Could you check a few things on this model? Use its own coordinates, in mm. Face numbers are marked on the shaded views. A direction names the side the tool comes from. Give positions to 0.01 mm unless a question says otherwise; leave off trailing zeros. Order: outer loops, then holes, each group sorted by start corner. A loop starts at its lowest first (then second) coordinate and runs counter-clockwise, first axis right, second up.
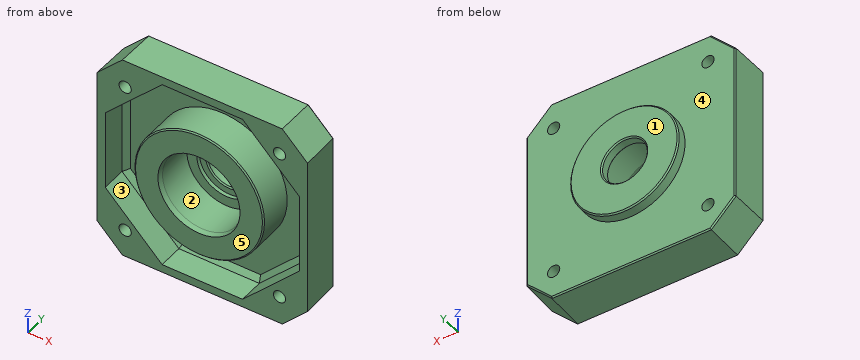
Autodesk Inventor part; units mm, degrees
ref_plane "YZ Plane" through (0, 0, 0) normal (1, 0, 0) x (0, 1, 0)
ref_plane "XZ Plane" through (0, 0, 0) normal (0, 1, 0) x (-1, 0, 0)
ref_plane "XY Plane" through (0, 0, 0) normal (0, 0, 1) x (1, 0, 0)
sketch "Sketch11" plane through (0, 0, 0) normal (0, 1, 0) x (-1, 0, 0)
  line L0 (-16, 21) -> (16, 21)
  line L1 (21, 16) -> (21, -16)
  line L2 (16, -21) -> (-16, -21)
  line L3 (-21, -16) -> (-21, 16)
  line L4 (-21, 21) -> (21, -21) construction
  line L5 (21, 21) -> (-21, -21) construction
  line L6 (21, -16) -> (16, -21)
  line L7 (-16, -21) -> (-21, -16)
  line L8 (-21, 16) -> (-16, 21)
  line L9 (16, 21) -> (21, 16)
  point P0 (0, 0)
  dimension "d82" = 42
  dimension "d83" = 5
  dimension "d84" = 5
  dimension "d85" = 5
  dimension "d86" = 5
  dimension "d87" = 5
  dimension "d88" = 5
  dimension "d89" = 5
  dimension "d90" = 5
extrude "Extrusion7" add sketch "Sketch11" against normal blind 8 draft 1
sketch "Sketch12" plane through (0, 0, 0) normal (0, 1, 0) x (1, 0, 0)
  circle A0 centre (0, 0) radius 10.9
  dimension "d93" = 21.8
extrude "Extrusion8" add sketch "Sketch12" along normal blind 2
sketch "Sketch13" plane through (0, -8, 0) normal (0, -1, 0) x (1, 0, 0)
  circle A0 centre (0, 0) radius 13
  line L0 (-8.0772, 19.5) -> (8.0772, 19.5)
  line L1 (8.0772, 19.5) -> (19.5, 8.0772)
  line L2 (19.5, 8.0772) -> (19.5, -8.0772)
  line L3 (19.5, -8.0772) -> (8.0772, -19.5)
  line L4 (8.0772, -19.5) -> (-8.0772, -19.5)
  line L5 (-8.0772, -19.5) -> (-19.5, -8.0772)
  line L6 (-19.5, -8.0772) -> (-19.5, 8.0772)
  line L7 (-19.5, 8.0772) -> (-8.0772, 19.5)
  dimension "d96" = 26
  dimension "d97" = 39
extrude "Extrusion9" cut sketch "Sketch13" against normal blind 6
sketch "Sketch14" plane through (0, -8, 0) normal (0, -1, 0) x (1, 0, 0)
  circle A0 centre (0, 0) radius 13
extrude "Extrusion10" add sketch "Sketch14" along normal blind 1
sketch "Sketch15" plane through (0, -9, 0) normal (0, -1, 0) x (1, 0, 0)
  circle A0 centre (0, 0) radius 8
  dimension "d102" = 16
extrude "Extrusion11" cut sketch "Sketch15" against normal blind 8.25
sketch "Sketch16" plane through (0, 2, 0) normal (0, 1, 0) x (1, 0, 0)
  point P0 (0, 0)
  point P1 (0, 0)
hole "Hole5" at (0, 2, 0) direction (0, -1, 0) diameter 9 end through all
sketch "Sketch17" plane through (0, -0.75, 0) normal (0, -1, 0) x (1, 0, 0)
  circle A0 centre (0, 0) radius 6
  dimension "d112" = 12
extrude "Extrusion12" cut sketch "Sketch17" against normal blind 0.75
sketch "Sketch18" plane through (0, 0, 0) normal (0, 1, 0) x (1, 0, 0)
  line L0 (-15.5, 15.5) -> (15.5, 15.5) construction
  line L1 (15.5, 15.5) -> (15.5, -15.5) construction
  line L2 (15.5, -15.5) -> (-15.5, -15.5) construction
  line L3 (-15.5, -15.5) -> (-15.5, 15.5) construction
  line L4 (-15.5, 15.5) -> (15.5, -15.5) construction
  line L5 (15.5, 15.5) -> (-15.5, -15.5) construction
  point P0 (0, 0)
  point P1 (0, 0)
  dimension "d115" = 31
  dimension "d124" = 31
hole "Hole6" at (-15.5, 0, -15.5) at (15.5, 0, -15.5) at (15.5, 0, 15.5) at (-15.5, 0, 15.5) direction (0, -1, 0) diameter 2.459 end through all
chamfer "Chamfer1" distance 0.25 distance2 1 1 edges at (-8, -9, 0) measured on face at (11.1299, -9, -1.6752)
chamfer "Chamfer2" distance 0.25 angle 45 12 edges at (-13, -9, 0) (0, 0, -4.5) (0, 2, -4.5) (-10.9, 2, 0) (-21, 0, 0) (-18.5, 0, 18.5) (0, 0, 21) (18.5, 0, 18.5) (21, 0, 0) (18.5, 0, -18.5) (0, 0, -21) (-18.5, 0, -18.5)
chamfer "Chamfer3" distance 1 angle 45 8 edges at (-13.7886, -2, -13.7886) (-19.5, -2, 0) (-13.7886, -2, 13.7886) (0, -2, 19.5) (13.7886, -2, 13.7886) (19.5, -2, 0) (13.7886, -2, -13.7886) (0, -2, -19.5)
equation "\"d84\" = d83"
equation "\"d85\" = d83"
equation "\"d86\" = d85"
equation "\"d87\" = d83"
equation "\"d88\" = d87"
equation "\"d89\" = d83"
equation "\"d90\" = d89"
properties part number "Nema 17 Top Cap" material "Aluminum 6061"
Item 1: For pin 1 (4 mm diameter, centred on x = -3.5, y = -2, fed in from +Z); pin 2 (1.5 mm diameter, centred on x = -8, y = -7, fed in from -Z); pin 3 (2 mm diameter, centred on x = 4.5, y = -0.5, fed in from -Z), each with a flat end and sliding along its axis, tell me the tip position at first contact or that it passes through.
Findings:
pin 1: stops at z = 21.07
pin 2: stops at z = -21.14
pin 3: stops at z = -21.03
Item 2: We'd pull the mould along Z, two halves only. Please class the marked faces 1 and 2: +Z half, -Z half, draft (parallel to the pull), parting line (faces both ways), or undercut.
Findings:
face 1: draft
face 2: undercut
Item 3: Imagine slicing it at B-B on y = -4. List the corners of the cut face in (x, z) for me.
Findings:
outline: (-21.07, -16.03) - (-16.03, -21.07) - (16.03, -21.07) - (21.07, -16.03) - (21.07, 16.03) - (16.03, 21.07) - (-16.03, 21.07) - (-21.07, 16.03) - close; circle Ø26 at (0, 0); hole (-19.5, -8.08) - (-8.08, -19.5) - (8.08, -19.5) - (19.5, -8.08) - (19.5, 8.08) - (8.08, 19.5) - (-8.08, 19.5) - (-19.5, 8.08) - close; hole circle Ø2.46 at (-15.5, -15.5); hole circle Ø2.46 at (-15.5, 15.5); hole circle Ø16 at (0, 0); hole circle Ø2.46 at (15.5, -15.5); hole circle Ø2.46 at (15.5, 15.5)
Item 4: Imagine slicing it at C-C on y = 1. List the corners of the cut face in (x, z) for me.
Findings:
outline: circle Ø21.8 at (0, 0); hole circle Ø9 at (0, 0)
Item 5: Please list where these lines run through material, in increasing order: line 1 along Z through (x, y) = (-15.5, -4.5); line 2 along X through (y, z) = (1.35, 0); line 3 along Z through (x, y) = (0, -0.5).
Findings:
line 1: z = -21.08 to -16.73, -14.27 to -12.08, 12.08 to 14.27, 16.73 to 21.08
line 2: x = -10.9 to -4.5, 4.5 to 10.9
line 3: z = -21.01 to -6, 6 to 21.01
Item 6: For the marked faces 3, 4 and 5, which set-ups out of +Z, -Z, +X, -X, +Y, -Y let a thin tool reach every point of the face, with its end or its side?
Findings:
face 3: -Y
face 4: +Y
face 5: +Z, -Z, +X, -X, -Y
Item 7: Imagine slicing it at A-A on y = -6.25. List the corners of the cut face in (x, z) for me, then the cut area to 3 significant figures.
Findings:
outline: (-21.11, -16.05) - (-16.05, -21.11) - (16.05, -21.11) - (21.11, -16.05) - (21.11, 16.05) - (16.05, 21.11) - (-16.05, 21.11) - (-21.11, 16.05) - close; circle Ø26 at (0, 0); hole (-19.5, -8.08) - (-8.08, -19.5) - (8.08, -19.5) - (19.5, -8.08) - (19.5, 8.08) - (8.08, 19.5) - (-8.08, 19.5) - (-19.5, 8.08) - close; hole circle Ø2.46 at (-15.5, -15.5); hole circle Ø2.46 at (-15.5, 15.5); hole circle Ø16 at (0, 0); hole circle Ø2.46 at (15.5, -15.5); hole circle Ø2.46 at (15.5, 15.5)
area: 782 mm2
